Drawing for the job (mm, zero at the part's lowest x, y, z). A direction names the side the tool comes from. Round coordinates to 2 decimals unless told otherwise and drop trailing zeros. Loops run counter-clockwise (first coordinate to the right, second up) from the corner with the lowest first, then second, coordinate; pieces in that order, holes last.
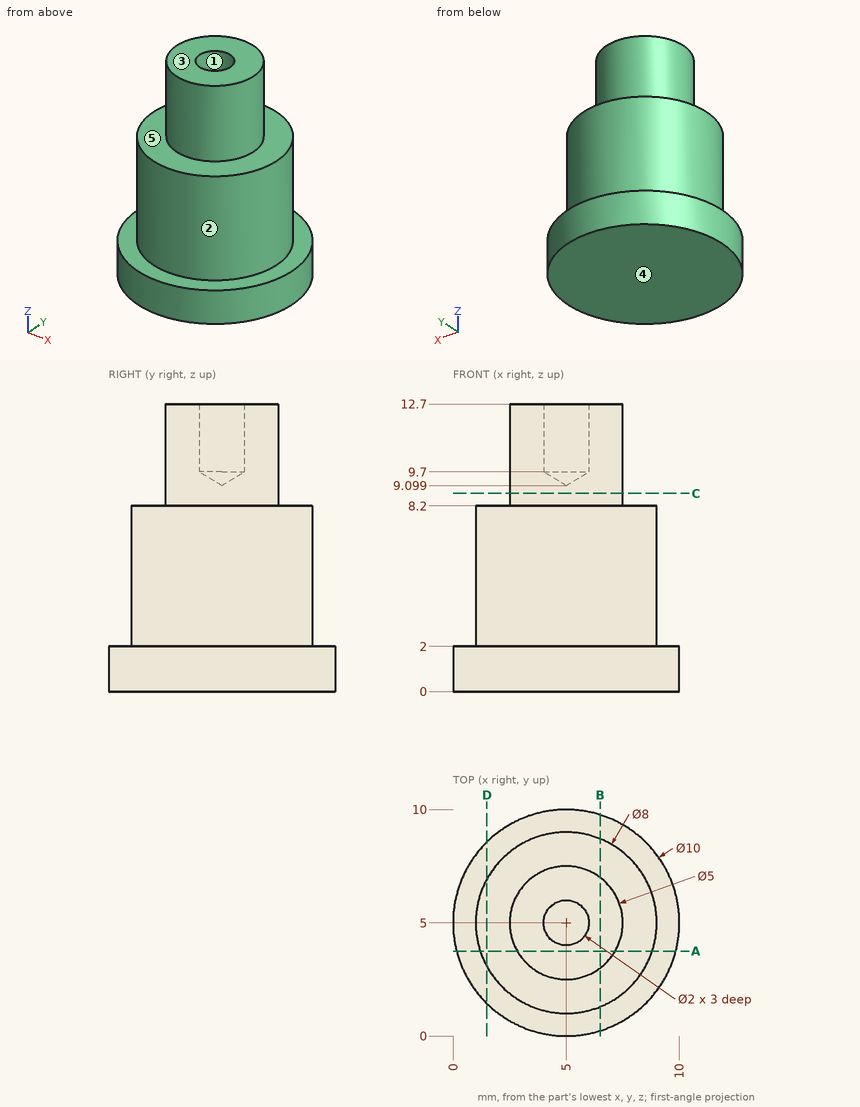
Q1. Flat gauge pins, fed straight in: P1, Ø1, axis at y = 9, z = 10, coming from the +X side; P2, Ø2, axis at y = 5, z = 4, coming from the +X side; P3, Ø1.5, axis at x = 6, z = 4, coming from the +Y side; P4, Ø5, axis at y = 8.5, z = 8.5, coming from the +X side. Where does each tip first touch, or does it go through?
Q2. Slice it at D-D on x = 1.5. Give the cut face in (y, z), plus the area to 3 significant figures.
Q3. Slice it at B-B on x = 6.5. Give the cut face in (y, z).
Q4. Tool access for the marked faces 4 and 5: list every direction of +Z, -Z, +X, -X, +Y, -Y with a clear straight run to the whole face (end or side of a thin tool).
Q5. Pull direction X, two halves, no side cores. Call the marked faces 1, 2 and 3: pulls with the +X half, pulls with the -X half, needs draft (parallel to the pull), parting line crosses it, or undercut.
Q6. Slice it at A-A on y = 3.75. Give the cut face in (x, z) (1 decimal).
Q7. Probe line 1 (Y direction, x = 5, z = 10.45); line 2 (Z direction, x = 1.5, y = 3.25); line 3 (Z direction, x = 8.75, y = 2). List the from-to ranges inside material, lowest first.
Q8. Slice it at C-C on z = 8.75. Give the cut face in (x, y), plus the area to 3 significant figures.
Reply:
1. P1: passes through
1. P2: stops at x = 9
1. P3: stops at y = 8.99
1. P4: stops at x = 8.87
2. outline: (1.43, 0) - (8.57, 0) - (8.57, 2) - (6.94, 2) - (6.94, 8.2) - (3.06, 8.2) - (3.06, 2) - (1.43, 2) - close
2. area: 38.3 mm2
3. outline: (0.23, 0) - (9.77, 0) - (9.77, 2) - (8.71, 2) - (8.71, 8.2) - (7, 8.2) - (7, 12.7) - (3, 12.7) - (3, 8.2) - (1.29, 8.2) - (1.29, 2) - (0.23, 2) - close
4. face 4: -Z, +X, -X, +Y, -Y
4. face 5: +Z
5. face 1: undercut
5. face 2: parting line crosses it
5. face 3: needs draft
6. outline: (0.2, 0) - (9.8, 0) - (9.8, 2) - (8.8, 2) - (8.8, 8.2) - (7.2, 8.2) - (7.2, 12.7) - (2.8, 12.7) - (2.8, 8.2) - (1.2, 8.2) - (1.2, 2) - (0.2, 2) - close
7. line 1: y = 2.5 to 4, 6 to 7.5
7. line 2: z = 0 to 8.2
7. line 3: z = 0 to 2
8. outline: circle Ø5 at (5, 5)
8. area: 19.6 mm2
